```python
from build123d import *


with BuildPart() as part:
    # Sketch1 → Revolução1 (revolve)
    with BuildSketch(Plane.XY, mode=Mode.PRIVATE) as revolu_o1_sk:
        with BuildLine():
            Line((1, 7.5), (12, 7.5))
            ThreePointArc((12, 7.5), (12.707106781, 7.792893219), (13, 8.5))
            Line((13, 8.5), (13, 11.85))
            Line((13, 11.85), (9.582687302, 11.85))
            ThreePointArc((9.582687302, 11.85), (6.5, 10.381), (3.417312698, 11.85))
            Line((3.417312698, 11.85), (0, 11.85))
            Line((0, 11.85), (0, 8.5))
            ThreePointArc((0, 8.5), (0.292893219, 7.792893219), (1, 7.5))
        make_face()
    revolve(revolu_o1_sk.sketch.rotate(Axis((50, 0, 0), (-1, 0, 0)), 270), axis=Axis((50, 0, 0), (-1, 0, 0)))


solid = part.part
```
The listing builds one solid part. Answer for the finished solid, in the listing's coordinates (mm). Give positions to 0.01 mm unless a question says otherwise; leave off trailing zeros. Order: outer loops, then holes, each group sorted by start corner. A loop starts at its lowest first (then second) coordinate and runs counter-clockwise, first axis right, second up.
1) Find section A-A on y = 0. Write down the section's boundary in (x, z), then the cut area to 3 significant figures.
Reported:
outline: (0, -11.85) - (3.42, -11.85) arc R3.97 cw to (9.58, -11.85) - (13, -11.85) - (13, -8.5) arc R1 ccw to (12, -7.5) - (1, -7.5) arc R1 ccw to (0, -8.5) - close; (0, 8.5) arc R1 ccw to (1, 7.5) - (12, 7.5) arc R1 ccw to (13, 8.5) - (13, 11.85) - (9.58, 11.85) arc R3.97 cw to (3.42, 11.85) - (0, 11.85) - close
area: 99.6 mm2
2) Consider line 1 along Y through (x, z) = (7.5, 6.75); line 2 along Z through (x, y) = (12, -2.25); line 3 along Y through (x, z) = (10.5, -1.75). Determine where each line is inside the solid, lowest interval first.
Reported:
line 1: y = -8.05 to -3.27, 3.27 to 8.05
line 2: z = -11.63 to -7.15, 7.15 to 11.63
line 3: y = -11.72 to -7.29, 7.29 to 11.72
3) Given P1, Ø1.5, axis at x = 9, y = 6.5, coming from the +Z side; P2, Ø6, axis at x = 9, z = -7.5, coming from the +Y side; P3, Ø5, axis at x = 8, z = -7, coming from the -Y side; P4, Ø9, axis at y = 0, z = 0, coming from the -X side (3 decimals), each flat-ended and moving along its own axis, determine where each tip first touches the part or whether it passes through.
Reported:
P1: stops at z = 10.2
P2: stops at y = 10.94
P3: stops at y = -10.71
P4: passes through
4) Find section C-C on x = 7. Write down the section's boundary in (y, z), then the cut area to 3 significant figures.
Reported:
outline: circle Ø20.83 at (0, 0); hole circle Ø15 at (0, 0)
area: 164 mm2
